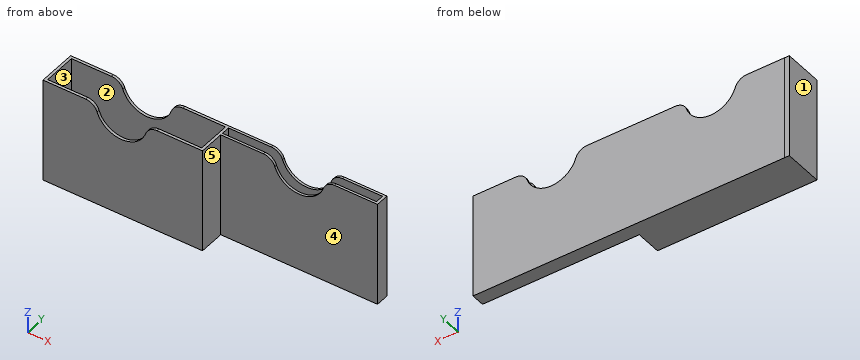
Autodesk Fusion 360 part; units mm, degrees
sketch "Sketch1" plane through (0, 0, 0) normal (0, 0, 1) x (1, 0, 0)
  line L0 (-48.6499, 24.8) -> (41.3501, 24.8)
  line L1 (40, 23.2) -> (40, 3.6)
  line L2 (40, 2) -> (-51.6764, 2)
  line L3 (-50, 3.6) -> (-50, 23.2)
  line L4 (-51.6, 24.7889) -> (-51.6, 2)
  line L5 (-51.6, 2) -> (-51.6764, 2)
  line L6 (-51.6, 24.7889) -> (-48.6499, 24.8)
  line L7 (41.3501, 24.8) -> (41.6, 24.8)
  line L8 (41.6, 2) -> (40, 2)
  line L9 (-50, 23.2) -> (40, 23.2)
  line L10 (-50, 3.6) -> (40, 3.6)
  line L11 (41.6, 17) -> (131.6, 17)
  line L12 (41.6, 18.4) -> (131.6, 18.4)
  line L13 (41.6, 24.8) -> (131.6, 24.8)
  line L14 (41.6, 23.4) -> (131.6, 23.4)
  line L15 (131.6, 18.4) -> (131.6, 23.4)
  line L16 (131.6, 24.8) -> (133.2, 24.8)
  line L17 (131.6, 17) -> (133.2, 17)
  line L18 (133.2, 17) -> (133.2, 24.8)
  line L19 (41.6, 23.4) -> (41.6, 18.4)
  line L20 (41.6, 17) -> (41.6, 2)
  dimension "d1" = 90
  dimension "d2" = 23
  dimension "d3" = 1.6
  dimension "d4" = 1.6
  dimension "d5" = 1.6
  dimension "d6" = 1.6
  dimension "d7" = 90
  dimension "d8" = 15
  dimension "d9" = 90
  dimension "d10" = 1.4
  dimension "d11" = 90
  dimension "d12" = 90
  dimension "d13" = 90
  dimension "d14" = 1.4
  dimension "d15" = 1.6
  dimension "d16" = 1.6
extrude "Extrude1" add sketch "Sketch1" along normal blind 61
extrude "Extrude2" add sketch "Sketch1" along normal blind 1 contours L1 L3 L9 L10 | L12 L14 L15 L19
sketch "Sketch2" plane through (0, 2, 0) normal (0, -1, 0) x (1, 0, 0)
  line L0 (-51.6, 0) -> (40, 0)
  line L1 (40, 0) -> (40, 61)
  line L2 (40, 61) -> (-51.6, 61)
  line L3 (-51.6, 61) -> (-51.6, 0)
  arc A0 (-20.8, 61) -> (9.2, 61) centre (-5.8, 61) ccw
  dimension "d21" = 30
sketch "Sketch3" plane through (0, 17, 0) normal (0, -1, 0) x (1, 0, 0)
  line L0 (41.6, 0) -> (133.2, 0)
  line L1 (133.2, 0) -> (133.2, 61)
  line L2 (133.2, 61) -> (41.6, 61)
  line L3 (41.6, 61) -> (41.6, 0)
  arc A0 (72.4, 61) -> (102.4, 61) centre (87.4, 61) ccw
  dimension "d22" = 30
extrude "Extrude3" cut sketch "Sketch2" against normal blind 41 contours L2 A0
extrude "Extrude4" cut sketch "Sketch3" against normal blind 28 contours L2 A0
fillet "Fillet1" radius 7 8 edges at (-20.8, 24, 61) (-20.8, 2.8, 61) (9.2, 2.8, 61) (9.2, 24, 61) (72.4, 24.1, 61) (72.4, 17.7, 61) (102.4, 17.7, 61) (102.4, 24.1, 61)
CAD build for the part. Positions are in the model's coordinates, mm. Face numbers are marked on the shaded views. A direction names the side the tool comes from. Round coordinates to 2 decimals unless told otherwise and drop trailing zeros. Write each loop counter-clockwise with the first axis right and the second up, starting at its lowest first coordinate (ties: lowest second). Pieces come first, ordered by that corner, then holes.
(1) Drop flat-ended pins along their axis: P1, Ø4, axis at x = -6, y = 5.5, coming from the +Z side; P2, Ø1.5, axis at x = 84.5, y = 21.5, coming from the +Z side; P3, Ø10, axis at y = 8.5, z = 27, coming from the +X side. Give the stop position or say it passes through.
(2) Mould opens along X. For the marked faces 3, 4 and 5 say: pulls with the +X half, pulls with the -X half, needs draft (parallel to the pull), parting line crosses it, or undercut.
(3) Slice it at B-B, the plane y = 10.25. Write the cut outline in (x, z).
(4) Slice it at D-D, the plane z = 51. Count the separate pieces of the cut face and the enclosed holes in it, and give its area (3 significant figures).
(5) Probe line 1 along X through (y, z) = (14.5, 47.5); line 2 along X through (y, z) = (17.5, 18); line 3 along Y through (x, z) = (25, 47). List the from-to ranges inside material, lowest first.
(6) Slice it at A-A, the plane z = 12.5. Write the cut outline in (x, y), and give its area (3 significant figures).
(7) 3-axis set-ups, long thin cutter, end or side, ignore diameter. For the marked faces 1 and 2: which of +Z, -Z, +X, -X, +Y, -Y reach the whole face in a straight line?
(8) Slice it at C-C, the plane x = -39.5. Write the cut outline in (y, z).
From the geometry:
1. P1: stops at z = 46.02
1. P2: stops at z = 1
1. P3: stops at x = 41.6
2. face 3: undercut
2. face 4: needs draft
2. face 5: pulls with the +X half
3. outline: (-51.6, 0) - (41.6, 0) - (41.6, 61) - (40, 61) - (40, 1) - (-50, 1) - (-50, 61) - (-51.6, 61) - close
4. separate pieces: 3
4. enclosed holes: 0
4. area: 491 mm2
5. line 1: x = -51.6 to -50, 40 to 41.6
5. line 2: x = -51.6 to -50, 40 to 133.2
5. line 3: y = 2 to 3.6, 23.2 to 24.8
6. outline: (-51.6, 2) - (41.6, 2) - (41.6, 17) - (133.2, 17) - (133.2, 24.8) - (-48.65, 24.8) - (-51.6, 24.79) - close; hole (-50, 3.6) - (40, 3.6) - (40, 23.2) - (-50, 23.2) - close; hole (41.6, 18.4) - (131.6, 18.4) - (131.6, 23.4) - (41.6, 23.4) - close
6. area: 625 mm2
7. face 1: +Z, -Z, -X, +Y, -Y
7. face 2: +Z
8. outline: (2, 0) - (24.8, 0) - (24.8, 61) - (23.2, 61) - (23.2, 1) - (3.6, 1) - (3.6, 61) - (2, 61) - close
